```python
from build123d import *

# Parameters (mm, degrees)
SKETCH1_W           = 1828.8
SKETCH1_H           = 863.6
BOSS_EXTRUDE1_DEPTH = 50.8
SKETCH2_W           = 1676.4
SKETCH2_H           = 711.2
SKETCH2_W_2         = 1600.2
SKETCH2_H_2         = 635
BOSS_EXTRUDE2_DEPTH = 50.8
SKETCH3_W           = 38.1
SKETCH3_H           = 38.1
BOSS_EXTRUDE3_DEPTH = 660.4
BOSS_EXTRUDE4_REACH = 1907.72
SKETCH4_W           = 38.1
SKETCH4_H           = 38.1
BOSS_EXTRUDE5_REACH = 1381.632
SKETCH5_W           = 38.1
SKETCH5_H           = 38.1


with BuildPart() as part:
    # Sketch1 → Boss-Extrude1 (new body)
    with BuildSketch(Plane(origin=(0, 0, 0), x_dir=(1, 0, 0), z_dir=(0, 1, 0))):
        Rectangle(SKETCH1_W, SKETCH1_H)
    extrude(amount=BOSS_EXTRUDE1_DEPTH)

    # Sketch2 → Boss-Extrude2 (add)
    with BuildSketch(Plane.XZ):
        Rectangle(SKETCH2_W, SKETCH2_H)
        Rectangle(SKETCH2_W_2, SKETCH2_H_2, mode=Mode.SUBTRACT)
    extrude(amount=BOSS_EXTRUDE2_DEPTH)

    # Sketch3 → Boss-Extrude3 (add)
    with BuildSketch(Plane.XZ.offset(50.8)):
        with Locations((-819.15, 336.55)):
            Rectangle(SKETCH3_W, SKETCH3_H)
        with Locations((819.15, 336.55)):
            Rectangle(SKETCH3_W, SKETCH3_H)
        with Locations((819.15, -336.55)):
            Rectangle(SKETCH3_W, SKETCH3_H)
        with Locations((-819.15, -336.55)):
            Rectangle(SKETCH3_W, SKETCH3_H)
    extrude(amount=BOSS_EXTRUDE3_DEPTH)

    # Sketch4 → Boss-Extrude4 (add, up to next)
    with BuildSketch(Plane(origin=(-800.1, 0, 0), x_dir=(0, 0, -1), z_dir=(1, 0, 0)), mode=Mode.PRIVATE) as boss_extrude4_sk1:
        with Locations((-336.55, -692.15)):
            Rectangle(SKETCH4_W, SKETCH4_H)
    boss_extrude4_tool1 = extrude(boss_extrude4_sk1.sketch, amount=BOSS_EXTRUDE4_REACH, mode=Mode.PRIVATE) - part.part
    # Sketch4 → Boss-Extrude4 (add, up to next)
    with BuildSketch(Plane(origin=(-800.1, 0, 0), x_dir=(0, 0, -1), z_dir=(1, 0, 0)), mode=Mode.PRIVATE) as boss_extrude4_sk2:
        with Locations((336.55, -692.15)):
            Rectangle(SKETCH4_W, SKETCH4_H)
    boss_extrude4_tool2 = extrude(boss_extrude4_sk2.sketch, amount=BOSS_EXTRUDE4_REACH, mode=Mode.PRIVATE) - part.part
    add(boss_extrude4_tool1.solids().sort_by_distance((-800.1, -692.15, 336.55))[0])
    add(boss_extrude4_tool2.solids().sort_by_distance((-800.1, -692.15, -336.55))[0])

    # Sketch5 → Boss-Extrude5 (add, up to next)
    with BuildSketch(Plane.XY.offset(-317.5), mode=Mode.PRIVATE) as boss_extrude5_sk1:
        with Locations((-819.15, -692.15)):
            Rectangle(SKETCH5_W, SKETCH5_H)
    boss_extrude5_tool1 = extrude(boss_extrude5_sk1.sketch, amount=BOSS_EXTRUDE5_REACH, mode=Mode.PRIVATE) - part.part
    # Sketch5 → Boss-Extrude5 (add, up to next)
    with BuildSketch(Plane.XY.offset(-317.5), mode=Mode.PRIVATE) as boss_extrude5_sk2:
        with Locations((819.15, -692.15)):
            Rectangle(SKETCH5_W, SKETCH5_H)
    boss_extrude5_tool2 = extrude(boss_extrude5_sk2.sketch, amount=BOSS_EXTRUDE5_REACH, mode=Mode.PRIVATE) - part.part
    add(boss_extrude5_tool1.solids().sort_by_distance((-819.15, -692.15, -317.5))[0])
    add(boss_extrude5_tool2.solids().sort_by_distance((819.15, -692.15, -317.5))[0])


solid = part.part
```
For this review, take the finished solid that the model builds, in its own axes (mm). A direction names the side the tool comes from. Round coordinates to 2 decimals unless told otherwise and drop trailing zeros. Write each loop counter-clockwise with the first axis right and the second up, starting at its lowest first coordinate (ties: lowest second). Pieces come first, ordered by that corner, then holes. Notation, with made-up numbers: (-3.75, 82.25) -> (50.25, 82.25) arc R23 ccw to (50.25, 119.25) -> close; hole circle Ø8 at (-10, 12). An arc over 180 degrees is marked (long way). One line per question, with ' | ' between items. Start each with the question number.
(1) Add section A-A, the plane x = 697.5. Write out the cut boundary in (y, z), plus the area to 3 significant figures.
(2) For line 1 along Z through (x, y) = (-564, -45); line 2 along X through (y, z) = (-545, 340.5); line 3 along Y through (x, z) = (-371, 30.5), list the stretches that pass through material, from the lowest coordinate up. Write a range as from..to.
(3) Mouldability with a two-part tool opening along Z and no side actions: class faces 1 (the face through (-4, -711.2, -318)), 2 (the face through (-11, -25, 317.5)), 3 (the face through (-13, 25, -431.8)) as released by +Z, released by -Z, zero draft, split by the parting line, or undercut.
(4) Tool access review of faces 4 (the face through (838.2, -357, -318)), 5 (the face through (-800.1, -358, -337)), 6 (the face through (-819, -366, -317.5)), 7 (the face through (-72, 0, 382)): name each direction out of +Z, -Z, +X, -X, +Y, -Y from which nothing blocks a thin tool from reaching the whole face with its end or side.
(5) Add section B-B, the plane z = -39. Write out the cut boundary in (x, y).
(6) Add section C-C, the plane y = -106.5. Write out the cut boundary in (x, z), plus the area to 3 significant figures.
(7) Insertion check: P1, Ø11.5, axis at y = -387.5, z = -338, coming from the -X side; P2, Ø19, axis at x = 45, y = -688, coming from the +Z side; P3, Ø8, axis at x = 374.5, z = -216.5, coming from the -Y side. Each pin has a flat end and moves straight along its axis. Give the tip position at first contact, or say it passes through.
Answer list:
1) outline: (-711.2, -355.6) -> (-673.1, -355.6) -> (-673.1, -317.5) -> (-711.2, -317.5) -> close; (-711.2, 317.5) -> (-673.1, 317.5) -> (-673.1, 355.6) -> (-711.2, 355.6) -> close; (-50.8, -355.6) -> (0, -355.6) -> (0, -431.8) -> (50.8, -431.8) -> (50.8, 431.8) -> (0, 431.8) -> (0, 355.6) -> (-50.8, 355.6) -> (-50.8, 317.5) -> (0, 317.5) -> (0, -317.5) -> (-50.8, -317.5) -> close | area: 50,600 mm²
2) line 1: -355.6..-317.5, 317.5..355.6 | line 2: -838.2..-800.1, 800.1..838.2 | line 3: 0..50.8
3) face 1: zero draft | face 2: undercut | face 3: released by -Z
4) face 4: +Z, -Z, +X, -Y | face 5: +Z, -Z | face 6: +X, -X | face 7: -Y
5) outline: (-914.4, 0) -> (-838.2, 0) -> (-838.2, -50.8) -> (-800.1, -50.8) -> (-800.1, 0) -> (800.1, 0) -> (800.1, -50.8) -> (838.2, -50.8) -> (838.2, 0) -> (914.4, 0) -> (914.4, 50.8) -> (-914.4, 50.8) -> close; (-838.2, -711.2) -> (-800.1, -711.2) -> (-800.1, -673.1) -> (-838.2, -673.1) -> close; (800.1, -711.2) -> (838.2, -711.2) -> (838.2, -673.1) -> (800.1, -673.1) -> close
6) outline: (-838.2, -355.6) -> (-800.1, -355.6) -> (-800.1, -317.5) -> (-838.2, -317.5) -> close; (-838.2, 317.5) -> (-800.1, 317.5) -> (-800.1, 355.6) -> (-838.2, 355.6) -> close; (800.1, -355.6) -> (838.2, -355.6) -> (838.2, -317.5) -> (800.1, -317.5) -> close; (800.1, 317.5) -> (838.2, 317.5) -> (838.2, 355.6) -> (800.1, 355.6) -> close | area: 5,810 mm²
7) P1: x = -838.2 | P2: z = 355.6 | P3: y = 0
